```python
from build123d import *

# Parameters (mm, degrees)
SKETCH1_W           = 95
SKETCH1_H           = 230
BOSS_EXTRUDE1_DEPTH = 899.573333333
SKETCH2_R           = 50
CUT_EXTRUDE1_DEPTH  = 1200
SKETCH5_R           = 50
CUT_EXTRUDE4_DEPTH  = 226
SCALE1_SCALE        = 0.75


with BuildPart() as part:
    # Sketch1 → Boss-Extrude1 (new body)
    with BuildSketch(Plane(origin=(0, 0, 0), x_dir=(1, 0, 0), z_dir=(0, 1, 0))):
        Rectangle(SKETCH1_W, SKETCH1_H)
    extrude(amount=BOSS_EXTRUDE1_DEPTH)

    # Sketch2 → Cut-Extrude1 (cut)
    with BuildSketch(Plane(origin=(47.5, 0, 0), x_dir=(0, 0, -1), z_dir=(1, 0, 0))):
        with Locations((0, 799.573333333)):
            Circle(SKETCH2_R)
    extrude(amount=-CUT_EXTRUDE1_DEPTH, mode=Mode.SUBTRACT)

    # Sketch5 → Cut-Extrude4 (cut)
    with BuildSketch(Plane(origin=(47.5, 0, 0), x_dir=(0, 0, -1), z_dir=(1, 0, 0))):
        with Locations((0, 100)):
            Circle(SKETCH5_R)
    extrude(amount=-CUT_EXTRUDE4_DEPTH, mode=Mode.SUBTRACT)


with BuildPart() as part_1:
    # Scale1: scaled about (0, 449.786666667, 0)
    add(part.part.scale(SCALE1_SCALE).moved(Location((0, 112.446666667, 0))))


solid = part_1.part
```
The listing builds one solid part. Answer for the finished solid, in the listing's coordinates (mm). Round coordinates to 2 decimals unless told otherwise and drop trailing zeros. Write each loop counter-clockwise with the first axis right and the second up, starting at its lowest first coordinate (ties: lowest second). Pieces come first, ordered by that corner, then holes. Notation, with made-up numbers: (44, 80) -> (50, 80) arc R17 ccw to (50, 89) -> close; hole circle Ø3 at (-38.75, 75.25). An arc over 180 degrees is marked (long way). Answer as a JSON object with one key per item and string values. Group by question number.
Q1. Determine the mould class of faces 1 (the face through (0, 445, -86.25)), 2 (the face through (0.499, 749.308, 4.882)), 3 (the face through (-35.625, 445, 1)) for opening direction Z: pulls with the +Z half, pulls with the -Z half, needs draft (parallel to the pull), parting line crosses it, or undercut.
Q2. Section C-C (z = 25.5) is taken. Write down the section's boundary in (x, y) (3 decimals), plus the area to 3 significant figures.
Q3. Section A-A (z = 0) is taken. Write down the section's boundary in (x, y) (3 decimals).
Q4. Section B-B (x = 4) is taken. Write down the section's boundary in (y, z), plus the area to 3 significant figures.
Q5. Straight lines are drawn through the part: line 1 along Y through (x, z) = (-11, 0); line 2 along Y through (x, z) = (-9, -10); line 3 along Z through (x, y) = (-28.5, 713). For each, find the intervals that lie inside material, in ascending order.
Check values:
{
 "1": {"face 1": "pulls with the -Z half", "face 2": "undercut", "face 3": "needs draft"},
 "2": {"outline": "(-35.625, 112.447) -> (35.625, 112.447) -> (35.625, 159.951) -> (-35.625, 159.951) -> close; (-35.625, 214.942) -> (35.625, 214.942) -> (35.625, 684.631) -> (-35.625, 684.631) -> close; (-35.625, 739.622) -> (35.625, 739.622) -> (35.625, 787.127) -> (-35.625, 787.127) -> close", "area": "40,200 mm^2"},
 "3": {"outline": "(-35.625, 112.447) -> (35.625, 112.447) -> (35.625, 149.947) -> (-35.625, 149.947) -> close; (-35.625, 224.947) -> (35.625, 224.947) -> (35.625, 674.627) -> (-35.625, 674.627) -> close; (-35.625, 749.627) -> (35.625, 749.627) -> (35.625, 787.127) -> (-35.625, 787.127) -> close"},
 "4": {"outline": "(112.45, -86.25) -> (787.13, -86.25) -> (787.13, 86.25) -> (112.45, 86.25) -> close; hole circle Ø75 at (187.45, 0); hole circle Ø75 at (712.13, 0)", "area": "108,000 mm^2"},
 "5": {"line 1": "112.45 to 149.95, 224.95 to 674.63, 749.63 to 787.13", "line 2": "112.45 to 151.3, 223.59 to 675.98, 748.27 to 787.13", "line 3": "-86.25 to -37.49, 37.49 to 86.25"}
}
